Here's how the part is built. I have some questions about the finished solid (model axes, mm). A direction names the side the tool comes from. Coordinates: 2 decimals unless noted, no trailing zeros. Loops run counter-clockwise (first coordinate to the right, second up) from the corner with the lowest first, then second, coordinate; pieces in that order, holes last. Notation, with made-up numbers: (0, -11.5) -> (22, -11.5) arc R29 ccw to (22, 24.5) -> close; hole circle Ø4 at (-30.5, 7). An arc over 180 degrees is marked (long way). Answer as a JSON object with one key per item and string values. Group by question number.
Q1. Thinking about a two-plate mould opening in Z: for faces 3 (the flat face through (-0.1, 0.4, -4.5)), 4 (the cylindrical face through (-5.05, -3.86, 4.63)), 5 (the cylindrical face through (-0.75, -3.94, 5.7)), which applies, released by +Z, released by -Z, zero draft, split by the parting line, or undercut?
Q2. I need wall thicknesses on line 1 (Z direction, x = 0, y = 0.15); line 2 (Z direction, x = 0, y = -6); line 3 (X direction, y = -7.5, z = 3.75). Which ranges of each line are inside material? Lowest first, please.
Q3. I want a section at B-B on z = 1. Write out the boundary of the cut face in (x, y).
Q4. I want a section at C-C on y = -3.25. Write out the boundary of the cut face in (x, z).
Q5. I'm going to push flat-ended pins straight in: pin 1 (6 mm diameter, centred on x = -2.5, z = -1, fed in from +Y); pin 2 (1.5 mm diameter, centred on x = -4, y = -1.5, fed in from +Z); pin 3 (1.5 mm diameter, centred on y = -2.5, z = 3.5, fed in from +X); pin 4 (6 mm diameter, centred on x = 1, z = 0.5, fed in from -Y). Where does each tip first touch, or does it pass through?
Q6. On a 3-axis mill with a long thin cutter (end or side, diameter ignored), from which of +Z, -Z, +X, -X, +Y, -Y can I reach the whole of each face in a straight line? I mean faces 1 (the cylindrical face through (-0.943, 0.197, -4.247)), 2 (the flat face through (-3.4, 0, 3)). Say none if no direction works.
Q7. I want a section at A-A on x = 0. Write out the boundary of the cut face in (y, z), then the cut area to 3 significant figures.
Q8. I want a section at D-D on z = 5.5. Write out the boundary of the cut face in (x, y).
```python
from build123d import *

# Parameters (mm, degrees)
F0_R     = 6.85
F0_R_2   = 5.75
F0_R_3   = 4.35
F1_DEPTH = 8
F2_DEPTH = 25
F3_DEPTH = 0.4


with BuildPart() as f1:
    # F0 (on Front) → F1 (new body)
    with BuildSketch(Plane.XZ):
        Circle(F0_R)
        Circle(F0_R_2, mode=Mode.SUBTRACT)
        Circle(F0_R_2)
        Circle(F0_R_3, mode=Mode.SUBTRACT)
        Circle(F0_R_3)
    extrude(amount=F1_DEPTH)

    # F0 (on Front) → F2 (cut)
    with BuildSketch(Plane.XZ):
        Circle(F0_R_2)
        Circle(F0_R_3, mode=Mode.SUBTRACT)
        Circle(F0_R_3)
    extrude(amount=F2_DEPTH, mode=Mode.SUBTRACT)

    # F0 (on Front) → F3 (join)
    with BuildSketch(Plane.XZ):
        Circle(F0_R)
        Circle(F0_R_2, mode=Mode.SUBTRACT)
        Circle(F0_R_2)
        Circle(F0_R_3, mode=Mode.SUBTRACT)
    extrude(amount=-F3_DEPTH)


solid = f1.part
```
Result set:
{
 "1": {"face 3": "zero draft", "face 4": "split by the parting line", "face 5": "undercut"},
 "2": {"line 1": "z = -6.85 to -4.35, 4.35 to 6.85", "line 2": "z = -6.85 to -5.75, 5.75 to 6.85", "line 3": "x = -5.73 to -4.36, 4.36 to 5.73"},
 "3": {"outline": "(-6.78, -8) -> (-5.66, -8) -> (-5.66, 0) -> (-4.23, 0) -> (-4.23, 0.4) -> (-6.78, 0.4) -> close; (4.23, 0) -> (5.66, 0) -> (5.66, -8) -> (6.78, -8) -> (6.78, 0.4) -> (4.23, 0.4) -> close"},
 "4": {"outline": "circle Ø13.7 at (0, 0); hole circle Ø11.5 at (0, 0)"},
 "5": {"pin 1": "stops at y = 0.4", "pin 2": "stops at z = 6.03", "pin 3": "stops at x = 6.27", "pin 4": "passes through"},
 "6": {"face 1": "+Y, -Y", "face 2": "-Y"},
 "7": {"outline": "(-8, -6.85) -> (0.4, -6.85) -> (0.4, -4.35) -> (0, -4.35) -> (0, -5.75) -> (-8, -5.75) -> close; (-8, 5.75) -> (0, 5.75) -> (0, 4.35) -> (0.4, 4.35) -> (0.4, 6.85) -> (-8, 6.85) -> close", "area": "19.6 mm²"},
 "8": {"outline": "(-4.08, -8) -> (-1.68, -8) -> (-1.68, 0) -> (1.68, 0) -> (1.68, -8) -> (4.08, -8) -> (4.08, 0.4) -> (-4.08, 0.4) -> close"}
}
